Autodesk Fusion 360 part; units mm, degrees
sketch "Esboço1" plane through (0, 0, 0) normal (0, 0, 1) x (1, 0, 0)
  circle A0 centre (100, 50) radius 36.5
  circle A1 centre (100, 50) radius 28.5
  dimension "d1" = 73
  dimension "d2" = 57
extrude "Extrusão1" add sketch "Esboço1" along normal blind 3.5
sketch "Esboço2" plane through (0, 0, 0) normal (0, 0, -1) x (1, 0, 0)
  circle A0 centre (100, -50) radius 28.5
  circle A1 centre (100, -50) radius 36.5
  circle A2 centre (100, -50) radius 32.5
  dimension "d5" = 65
extrude "Extrusão2" add sketch "Esboço2" along normal blind 4 contours A2
sketch "Esboço3" plane through (0, 0, -4) normal (0, 0, -1) x (1, 0, 0)
  circle A0 centre (100, -50) radius 28.5
  circle A1 centre (100, -50) radius 32.5
  line L0 (55, -50) -> (160, -50) construction
  circle A2 centre (69.4606, -50) radius 1.5
  dimension "d8" = 3
extrude "Extrusão3" add sketch "Esboço3" along normal blind 4 contours A2
chamfer "Chanfro1" distance 1 angle 45 2 edges at (65.9701, 36.801, 0) (65.9701, 36.801, 3.5)
chamfer "Chanfro2" distance 0.5 angle 45 1 edges at (68.0621, 50.5424, -8)
Geometry: final body of the model. Coordinates: model frame, mm. A direction names the side the tool comes from. Round coordinates to 2 decimals unless told otherwise and drop trailing zeros. Order: outer loops, then holes, each group sorted by start corner. A loop starts at its lowest first (then second) coordinate and runs counter-clockwise, first axis right, second up. Notation, with made-up numbers: M 37,85 L 47,85 A11 ccw 47,96 Z; hole C 7,-15.75 d6. An arc over 180 degrees is marked long. Use one line per item in the form item = value. Start each with the question number.
Q1. Pin query (flat end, axial travel): pin 1 Ø1 at (y, z) = (74, -3) entering from -X; pin 2 Ø12 at (x, y) = (119, 61) entering from -Z; pin 3 Ø3 at (y, z) = (53, -3) entering from -X; pin 4 Ø1.5 at (y, z) = (42, -3.5) entering from -X. Return the tip coordinate at first contact, or that it passes through.
Q2. Cut plane C-C (z = -5). Return loops of the section in (x, y).
Q3. Cut plane B-B (x = 100). Return loops of the section in (y, z).
Q4. Access query for faces 4 (the face through (116, 21, 0)), 5 (the face through (134.814, 39.036, 1.74)). Directions: +Z, -Z, +X, -X, +Y, -Y. A direction counts if a zero-diameter tool reaches every point of the face in a straight line with its end or side. Return the directions, or none.
Q5. Material intervals for line 1 (Y direction, x = 100, z = 1.5); line 2 (Y direction, x = 100, z = -1); line 3 (X direction, y = 50.5, z = 1.5), sorted ascending. Write a range as [from, to].
Q6. Cut plane A-A (y = 50). Return loops of the section in (x, z), and give its area (4 significant figures).
Q7. Mould query, pull axis Y, two halves, no side actions, for faces 1 (the face through (69, 50, -8)), 2 (the face through (78.994, 30.738, -0.303)), 3 (the face through (67.53, 51.43, -1.97)). Classes: +Y half, -Y half, draft (parallel to the pull), parting line (faces both ways), or undercut.
Geometry results:
q1.pin_1 = 77.55
q1.pin_2 = through
q1.pin_3 = 67.53
q1.pin_4 = 68.32
q2.outline = C 69.46,50 d3
q3.outline = M 13.5,1 L 14.5,0 L 17.5,0 L 17.5,-4 L 21.5,-4 L 21.5,3.5 L 14.5,3.5 L 13.5,2.5 Z; M 78.5,-4 L 82.5,-4 L 82.5,0 L 85.5,0 L 86.5,1 L 86.5,2.5 L 85.5,3.5 L 78.5,3.5 Z
q4.face_4 = -Z
q4.face_5 = +Z, -Z
q5.line_1 = [13.5, 21.5], [78.5, 86.5]
q5.line_2 = [17.5, 21.5], [78.5, 82.5]
q5.line_3 = [63.5, 71.5], [128.5, 136.5]
q6.outline = M 63.5,1 L 64.5,0 L 67.5,0 L 67.5,-4 L 67.96,-4 L 67.96,-7.5 L 68.46,-8 L 70.46,-8 L 70.96,-7.5 L 70.96,-4 L 71.5,-4 L 71.5,3.5 L 64.5,3.5 L 63.5,2.5 Z; M 128.5,-4 L 132.5,-4 L 132.5,0 L 135.5,0 L 136.5,1 L 136.5,2.5 L 135.5,3.5 L 128.5,3.5 Z
q6.area = 97.75 mm^2
q7.face_1 = draft
q7.face_2 = undercut
q7.face_3 = parting line
